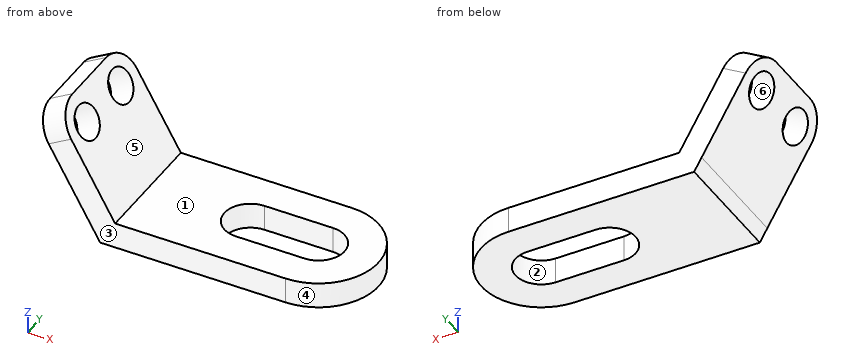
from build123d import *

# Parameters (mm, degrees)
F2_R     = 6.35
F3_DEPTH = 9.652
F4_DEPTH = 9.652
F6_DEPTH = 44.704


with BuildPart() as f3:
    # F2 (on face) → F3 (new body)
    with BuildSketch(Plane(origin=(-47.391302, 0, -27.361381), x_dir=(0, 1, 0), z_dir=(0.866025, 0, 0.5))):
        with BuildLine():
            Line((-22.352, 64.360201), (-22.352, 31.594201))
            Line((-22.352, 31.594201), (22.352, 31.594201))
            Line((22.352, 31.594201), (22.352, 64.360201))
            ThreePointArc((22.352, 64.360201), (19.15302, 72.083222), (11.43, 75.282201))
            Line((11.43, 75.282201), (-11.43, 75.282201))
            ThreePointArc((-11.43, 75.282201), (-19.15302, 72.083222), (-22.352, 64.360201))
        make_face()
        with Locations((-11.43, 64.360201)):
            Circle(F2_R, mode=Mode.SUBTRACT)
        with Locations((11.43, 64.360201)):
            Circle(F2_R, mode=Mode.SUBTRACT)
    extrude(amount=-F3_DEPTH)



with BuildPart() as f4:
    # F0 (on Top) → F4 (new body)
    with BuildSketch(Plane.XY):
        with BuildLine():
            Line((-63.188403, -22.352), (0.311597, -22.352))
            ThreePointArc((0.311597, -22.352), (22.663597, 0), (0.311597, 22.352))
            Line((0.311597, 22.352), (-63.188403, 22.352))
            Line((-63.188403, 22.352), (-63.188403, -22.352))
        make_face()
        with BuildLine():
            ThreePointArc((0.311597, 9.652), (9.963597, 0), (0.311597, -9.652))
            Line((0.311597, -9.652), (-25.088403, -9.652))
            ThreePointArc((-25.088403, -9.652), (-34.740403, 0), (-25.088403, 9.652))
            Line((-25.088403, 9.652), (0.311597, 9.652))
        make_face(mode=Mode.SUBTRACT)
    extrude(amount=-F4_DEPTH)


with BuildPart() as f3_1:
    add(f3.part)

    add(f4.part)  # F6 merges F4
    # F5 (on face) → F6 (join)
    with BuildSketch(Plane.XZ.offset(22.352)):
        Polygon((-63.188403, 0), (-71.54728, -4.826), (-68.760988, -9.652), (-63.188403, -9.652), align=None)
    extrude(amount=-F6_DEPTH)


solid = f3_1.part
Design review of the part built by this model. Coordinates are the model's own, in mm. Face numbers are marked on the shaded views. A direction names the side the tool comes from. Give positions to 0.01 mm unless a question says otherwise; leave off trailing zeros. Write each loop counter-clockwise with the first axis right and the second up, starting at its lowest first coordinate (ties: lowest second). Pieces come first, ordered by that corner, then holes. Notation, with made-up numbers: M 59,35.25 L 85,35.25 A16 cw 85,39.25 Z; hole C 15.25,-26 d10. An arc over 180 degrees is marked long. Return JSON: item names as keys, results as strings. Group by question number.
Item 1: Clearance check with flat-ended pins moving along their axes: pin 1 Ø4 at (y, z) = (3.5, -4.5) entering from -X; pin 2 Ø12 at (x, y) = (-66, -10) entering from +Z; pin 3 Ø4 at (x, y) = (-21.5, -16.5) entering from +Z. State where each tip first meets the part, or that it passes through.
Item 2: Take a section at C-C (z = 25). Count the separate pieces of the cut face and the enclosed holes in it, plus the area to 3 significant figures.
Item 3: Wall thickness on line 1 along Z through (x, y) = (-61.5, -12); line 2 along Z through (x, y) = (-71, -17.5); line 3 along Y through (x, z) = (2.5, -2): over which ranges is each line inside the solid? List them lowest first.
Item 4: Take a section at D-D (x = -38.5). Give the boundary of the cut face in (y, z).
Item 5: The part is to be moulded in two halves that separate along Z. For the marked faces 4, 5 and 6, say which applies: pulls with the +Z half, pulls with the -Z half, needs draft (parallel to the pull), parting line crosses it, or undercut.
Item 6: Take a section at B-B (z = -1.5). Give the boundary of the cut face in (x, y), plus the area to 3 significant figures.
Item 7: Tool access review of the marked faces 1, 2 and 3: name each direction out of +Z, -Z, +X, -X, +Y, -Y from which nothing blocks a thin tool from reaching the whole face with its end or side.
Return value:
{
 "1": {"pin 1": "stops at x = -72.89", "pin 2": "stops at z = 15.26", "pin 3": "stops at z = 0"},
 "2": {"separate pieces": "3", "enclosed holes": "0", "area": "229 mm2"},
 "3": {"line 1": "z = -9.65 to 0", "line 2": "z = -5.77 to 13.53", "line 3": "y = -22.24 to -9.4, 9.4 to 22.24"},
 "4": {"outline": "M -22.35,-9.65 L 22.35,-9.65 L 22.35,0 L -22.35,0 Z"},
 "5": {"face 4": "needs draft", "face 5": "pulls with the +Z half", "face 6": "undercut"},
 "6": {"outline": "M -73.47,-22.35 L 0.31,-22.35 A22.35 ccw 0.31,22.35 L -73.47,22.35 Z; hole M -25.09,-9.65 L 0.31,-9.65 A9.65 ccw 0.31,9.65 L -25.09,9.65 A9.65 ccw Z", "area": "3,300 mm2"},
 "7": {"face 1": "+Z, +X, +Y, -Y", "face 2": "+Z, -Z", "face 3": "+Z, -Z, +X, -X, -Y"}
}
